Build history of the part. All positions in model axes, mm. A direction names the side the tool comes from. Coordinates: 2 decimals unless noted, no trailing zeros. One line per item, written item: value.
from build123d import *

# Parameters (mm, degrees)
BR_EXTRUDE_DEPTH      = 280
BR_EXTRUDE_DEPTH_BACK = 280


with BuildPart() as part:
    # Sketch2 → BR_Extrude (new body, two sides)
    with BuildSketch(Plane(origin=(0, 0, 0), x_dir=(0, 0, -1), z_dir=(1, 0, 0))) as br_extrude_sk:
        with BuildLine():
            Line((-10.05, 11.464213562), (-10.05, 14))
            Line((-10.05, 14), (-5, 14))
            Line((-5, 14), (-5, 18.5))
            Line((-5, 18.5), (-5.8, 18.5))
            Line((-5.8, 18.5), (-5.8, 20))
            Line((-5.8, 20), (-17, 20))
            ThreePointArc((-17, 20), (-19.121320344, 19.121320344), (-20, 17))
            Line((-20, 17), (-20, 5.8))
            Line((-20, 5.8), (-18.5, 5.8))
            Line((-18.5, 5.8), (-18.5, 5))
            Line((-18.5, 5), (-14, 5))
            Line((-14, 5), (-14, 10.05))
            Line((-14, 10.05), (-11.464213562, 10.05))
            Line((-11.464213562, 10.05), (-7.5, 6.085786438))
            Line((-7.5, 6.085786438), (-7.5, -6.085786438))
            Line((-7.5, -6.085786438), (-11.464213562, -10.05))
            Line((-11.464213562, -10.05), (-14, -10.05))
            Line((-14, -10.05), (-14, -5))
            Line((-14, -5), (-18.5, -5))
            Line((-18.5, -5), (-18.5, -5.8))
            Line((-18.5, -5.8), (-20, -5.8))
            Line((-20, -5.8), (-20, -17))
            ThreePointArc((-20, -17), (-19.121320344, -19.121320344), (-17, -20))
            Line((-17, -20), (-5.8, -20))
            Line((-5.8, -20), (-5.8, -18.5))
            Line((-5.8, -18.5), (-5, -18.5))
            Line((-5, -18.5), (-5, -14))
            Line((-5, -14), (-10.05, -14))
            Line((-10.05, -14), (-10.05, -11.464213562))
            Line((-10.05, -11.464213562), (-6.085786438, -7.5))
            Line((-6.085786438, -7.5), (6.085786438, -7.5))
            Line((6.085786438, -7.5), (10.05, -11.464213562))
            Line((10.05, -11.464213562), (10.05, -14))
            Line((10.05, -14), (5, -14))
            Line((5, -14), (5, -18.5))
            Line((5, -18.5), (5.8, -18.5))
            Line((5.8, -18.5), (5.8, -20))
            Line((5.8, -20), (17, -20))
            ThreePointArc((17, -20), (19.121320344, -19.121320344), (20, -17))
            Line((20, -17), (20, -5.8))
            Line((20, -5.8), (18.5, -5.8))
            Line((18.5, -5.8), (18.5, -5))
            Line((18.5, -5), (14, -5))
            Line((14, -5), (14, -10.05))
            Line((14, -10.05), (11.464213562, -10.05))
            Line((11.464213562, -10.05), (7.5, -6.085786438))
            Line((7.5, -6.085786438), (7.5, 6.085786438))
            Line((7.5, 6.085786438), (11.464213562, 10.05))
            Line((11.464213562, 10.05), (14, 10.05))
            Line((14, 10.05), (14, 5))
            Line((14, 5), (18.5, 5))
            Line((18.5, 5), (18.5, 5.8))
            Line((18.5, 5.8), (20, 5.8))
            Line((20, 5.8), (20, 17))
            ThreePointArc((20, 17), (19.121320344, 19.121320344), (17, 20))
            Line((17, 20), (5.8, 20))
            Line((5.8, 20), (5.8, 18.5))
            Line((5.8, 18.5), (5, 18.5))
            Line((5, 18.5), (5, 14))
            Line((5, 14), (10.05, 14))
            Line((10.05, 14), (10.05, 11.464213562))
            Line((10.05, 11.464213562), (6.085786438, 7.5))
            Line((6.085786438, 7.5), (-6.085786438, 7.5))
            Line((-6.085786438, 7.5), (-10.05, 11.464213562))
        make_face()
        with BuildLine():
            Line((8, 15.5), (8, 18.5))
            Line((8, 18.5), (14.5, 18.5))
            Line((14.5, 18.5), (14.5, 17.25))
            ThreePointArc((14.5, 17.25), (16.444543648, 16.444543648), (17.25, 14.5))
            Line((17.25, 14.5), (18.5, 14.5))
            Line((18.5, 14.5), (18.5, 8))
            Line((18.5, 8), (15.5, 8))
            Line((15.5, 8), (15.5, 11.75))
            Line((15.5, 11.75), (14.5, 11.75))
            ThreePointArc((14.5, 11.75), (12.555456352, 12.555456352), (11.75, 14.5))
            Line((11.75, 14.5), (11.75, 15.5))
            Line((11.75, 15.5), (8, 15.5))
        make_face(mode=Mode.SUBTRACT)
        with BuildLine():
            Line((8, -15.5), (11.75, -15.5))
            Line((11.75, -15.5), (11.75, -14.5))
            ThreePointArc((11.75, -14.5), (12.555456352, -12.555456352), (14.5, -11.75))
            Line((14.5, -11.75), (15.5, -11.75))
            Line((15.5, -11.75), (15.5, -8))
            Line((15.5, -8), (18.5, -8))
            Line((18.5, -8), (18.5, -14.5))
            Line((18.5, -14.5), (17.25, -14.5))
            ThreePointArc((17.25, -14.5), (16.444543648, -16.444543648), (14.5, -17.25))
            Line((14.5, -17.25), (14.5, -18.5))
            Line((14.5, -18.5), (8, -18.5))
            Line((8, -18.5), (8, -15.5))
        make_face(mode=Mode.SUBTRACT)
        with BuildLine():
            Line((-15.5, 8), (-18.5, 8))
            Line((-18.5, 8), (-18.5, 14.5))
            Line((-18.5, 14.5), (-17.25, 14.5))
            ThreePointArc((-17.25, 14.5), (-16.444543648, 16.444543648), (-14.5, 17.25))
            Line((-14.5, 17.25), (-14.5, 18.5))
            Line((-14.5, 18.5), (-8, 18.5))
            Line((-8, 18.5), (-8, 15.5))
            Line((-8, 15.5), (-11.75, 15.5))
            Line((-11.75, 15.5), (-11.75, 14.5))
            ThreePointArc((-11.75, 14.5), (-12.555456352, 12.555456352), (-14.5, 11.75))
            Line((-14.5, 11.75), (-15.5, 11.75))
            Line((-15.5, 11.75), (-15.5, 8))
        make_face(mode=Mode.SUBTRACT)
        with BuildLine():
            Line((-11.75, -14.5), (-11.75, -15.5))
            Line((-11.75, -15.5), (-8, -15.5))
            Line((-8, -15.5), (-8, -18.5))
            Line((-8, -18.5), (-14.5, -18.5))
            Line((-14.5, -18.5), (-14.5, -17.25))
            ThreePointArc((-14.5, -17.25), (-16.444543648, -16.444543648), (-17.25, -14.5))
            Line((-17.25, -14.5), (-18.5, -14.5))
            Line((-18.5, -14.5), (-18.5, -8))
            Line((-18.5, -8), (-15.5, -8))
            Line((-15.5, -8), (-15.5, -11.75))
            Line((-15.5, -11.75), (-14.5, -11.75))
            ThreePointArc((-14.5, -11.75), (-12.555456352, -12.555456352), (-11.75, -14.5))
        make_face(mode=Mode.SUBTRACT)
        with BuildLine():
            Line((-5.2, -5.2), (-5.2, -2.26102435))
            Line((-5.2, -2.26102435), (-4.585300372, -1.993745345))
            ThreePointArc((-4.585300372, -1.993745345), (-5, 0), (-4.585300372, 1.993745345))
            Line((-4.585300372, 1.993745345), (-5.2, 2.26102435))
            Line((-5.2, 2.26102435), (-5.2, 5.2))
            Line((-5.2, 5.2), (-2.26102435, 5.2))
            Line((-2.26102435, 5.2), (-1.993745345, 4.585300372))
            ThreePointArc((-1.993745345, 4.585300372), (0, 5), (1.993745345, 4.585300372))
            Line((1.993745345, 4.585300372), (2.26102435, 5.2))
            Line((2.26102435, 5.2), (5.2, 5.2))
            Line((5.2, 5.2), (5.2, 2.26102435))
            Line((5.2, 2.26102435), (4.585300372, 1.993745345))
            ThreePointArc((4.585300372, 1.993745345), (5, 0), (4.585300372, -1.993745345))
            Line((4.585300372, -1.993745345), (5.2, -2.26102435))
            Line((5.2, -2.26102435), (5.2, -5.2))
            Line((5.2, -5.2), (2.26102435, -5.2))
            Line((2.26102435, -5.2), (1.993745345, -4.585300372))
            ThreePointArc((1.993745345, -4.585300372), (0, -5), (-1.993745345, -4.585300372))
            Line((-1.993745345, -4.585300372), (-2.26102435, -5.2))
            Line((-2.26102435, -5.2), (-5.2, -5.2))
        make_face(mode=Mode.SUBTRACT)
    extrude(amount=BR_EXTRUDE_DEPTH)
    extrude(br_extrude_sk.sketch, amount=-BR_EXTRUDE_DEPTH_BACK)


solid = part.part
1. Two-plate mould, pull along Y, no slides. Class faces 1 (the face through (280, -6, 0)), 2 (the face through (4, -20, -11)), 3 (the face through (4, 0, -7.5)): pulls with the +Y half, pulls with the -Y half, needs draft (parallel to the pull), parting line crosses it, or undercut.
Values found:
face 1: needs draft
face 2: pulls with the -Y half
face 3: undercut
2. Flat gauge pins, fed straight in: P1, Ø10, axis at y = 10.5, z = 2, coming from the +X side; P2, Ø1.4, axis at x = 85, y = -18, coming from the -Z side; P3, Ø0.6, axis at x = -29, z = 5, coming from the +Y side; P4, Ø3, axis at x = -100, z = 4, coming from the -Y side. Where does each tip first touch, or does it go through?
Values found:
P1: stops at x = 280
P2: stops at z = -19.98
P3: stops at y = 18.5
P4: stops at y = -18.5
3. 3-axis set-ups, long thin cutter, end or side, ignore diameter. For faces 4 (the face through (4, 11, -20)), 5 (the face through (4, -7.5, 0)): which of +Z, -Z, +X, -X, +Y, -Y reach the whole face in a straight line?
Values found:
face 4: -Z, +X, -X, +Y, -Y
face 5: +X, -X
4. Probe line 1 along Y through (x, z) = (191, 11.5); line 2 along Y through (x, z) = (4, 4); line 3 along Z through (x, y) = (138, -5.5). List the from-to ranges inside material, lowest first.
Values found:
line 1: y = -20 to -18.5, -15.5 to -10.05, 10.05 to 15.5, 18.5 to 20
line 2: y = -7.5 to -5.2, 5.2 to 7.5
line 3: z = -18.5 to -14, -7.5 to 7.5, 14 to 18.5
5. Band-saw the part on A-A, the plane x = -235.5. Count the separate pieces of the cut face and the enclosed holes in it, and give its area (3 significant figures).
Values found:
separate pieces: 1
enclosed holes: 5
area: 555 mm2
